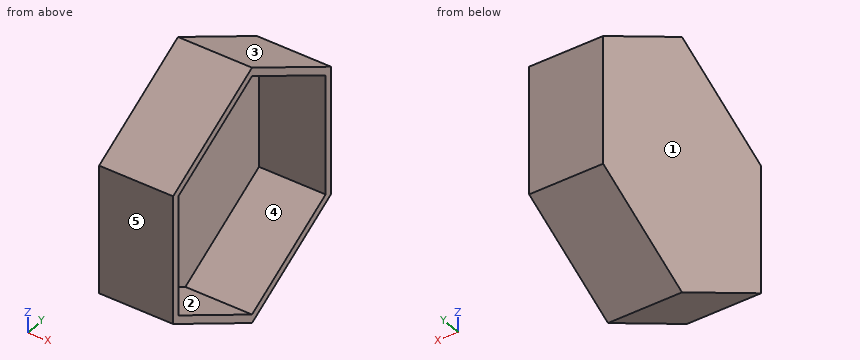
from build123d import *

# Parameters (mm, degrees)
RESSALTO_EXTRUS_O1_DEPTH = 50
CASCA1_T                 = -10


with BuildPart() as part:
    # Esboço1 → Ressalto-extrusão1 (new body, symmetric)
    with BuildSketch(Plane(origin=(0, 0, 0), x_dir=(0, 0, -1), z_dir=(1, 0, 0))):
        Polygon((173.205080757, 0), (86.602540378, 150), (-86.602540378, 150), (-173.205080757, 0), (-86.602540378, -150), (86.602540378, -150), align=None)
    extrude(amount=RESSALTO_EXTRUS_O1_DEPTH, both=True)

    # Casca1
    casca1_openings = [part.faces().sort_by_distance(p)[0] for p in [
        (50, 0, 0),
    ]]
    offset(amount=CASCA1_T, openings=casca1_openings, kind=Kind.INTERSECTION)


solid = part.part
Read the model definition and answer for the solid it produces. Units are mm, in the model's axes. Face numbers are marked on the shaded views. A direction names the side the tool comes from. Round coordinates to 2 decimals unless told otherwise and drop trailing zeros. Loops run counter-clockwise (first coordinate to the right, second up) from the corner with the lowest first, then second, coordinate; pieces in that order, holes last.
Q1. Each of these flat-tipped pins is pushed along its axis until it touches: pin 1 (4 mm diameter, centred on x = 15, y = -76.5, fed in from +Z); pin 2 (8 mm diameter, centred on y = -115, z = -34.5, fed in from +X); pin 3 (8 mm diameter, centred on x = 32, y = 73.5, fed in from +Z). Where does it stop, or does it pass through?
Q2. Determine the mould class of the marked faces 1, 2 and 3 for opening direction Y: released by +Y, released by -Y, zero draft, split by the parting line, or undercut.
Q3. Section A-A on x = 37 is taken. Write down the section's boundary in (y, z).
Q4. Section C-C on y = 37 is taken. Write down the section's boundary in (x, z), and give its area (3 significant figures).
Q5. Which of the six approach directions +Z, -Z, +X, -X, +Y, -Y give full straight-line access (tool end or side, diameter ignored) to the marked faces 4 and 5?
Q6. Section B-B on z = 45 is taken. Write down the section's boundary in (x, y), and give its area (3 significant figures).
Q7. Consider probe 1 along Y at (x, z) = (9, -79.5); probe 2 along X at (y, z) = (38.5, 94); probe 3 along Z at (x, y) = (-35, -53). Determine where each line is inside the solid, lowest interval first.
Output:
1. pin 1: stops at z = 130.19
1. pin 2: stops at x = -40
1. pin 3: stops at z = 133.08
2. face 1: zero draft
2. face 2: undercut
2. face 3: released by +Y
3. outline: (-150, -86.6) - (0, -173.21) - (150, -86.6) - (150, 86.6) - (0, 173.21) - (-150, 86.6) - close; hole (-140, -80.83) - (0, -161.66) - (140, -80.83) - (140, 80.83) - (0, 161.66) - (-140, 80.83) - close
4. outline: (-50, -151.84) - (50, -151.84) - (50, -140.3) - (-40, -140.3) - (-40, 140.3) - (50, 140.3) - (50, 151.84) - (-50, 151.84) - close
4. area: 5,120 mm2
5. face 4: +X
5. face 5: +Z, -Z, +X, -X, -Y
6. outline: (-50, -150) - (50, -150) - (50, -140) - (-40, -140) - (-40, 140) - (50, 140) - (50, 150) - (-50, 150) - close
6. area: 4,800 mm2
7. probe 1: y = -150 to -140, 140 to 150
7. probe 2: x = -50 to -40
7. probe 3: z = -142.61 to -131.06, 131.06 to 142.61
